Geometry check sheet. Reference: the model listing, model coordinates, mm. A direction names the side the tool comes from. Coordinates: 2 decimals unless noted, no trailing zeros. Loops run counter-clockwise (first coordinate to the right, second up) from the corner with the lowest first, then second, coordinate; pieces in that order, holes last. Notation, with made-up numbers: (-7.5, 81) - (47.5, 81) arc R19 ccw to (47.5, 92) - close; hole circle Ø9 at (4, -9). An arc over 180 degrees is marked (long way). Write each question's results on one line, items separated by ' | '. Start each with the question number.
(1) Material ranges on probe 1 along Y at (x, z) = (0, 6); probe 2 along Y at (x, z) = (0.5, 10.25); probe 3 along X at (y, z) = (-8, 2), recorded low to high.
(2) Sectioned sample at A-A (y = 0). Enter the section's corners in (x, z).
(3) Sectioned sample at B-B (x = 0). Enter the section's corners in (y, z).
(4) Mould release check, pull along X, two halves, no side actions. Record for faces 3 (the face through (10.4, -1.2, 5.6)), 4 (the face through (-6, 17, 0.95)), 5 (the face through (4.119, 18.548, 0.468)): pulls with the +X half, pulls with the -X half, needs draft (parallel to the pull), parting line crosses it, or undercut.
(5) Access from +Z, -Z, +X, -X, +Y, -Y to the whole of each face (thin tool, end or side, straight path). Record for faces 1 (the face through (12.384, 5.419, 5.552)), 2 (the face through (-13.887, -10.648, 5.88)).
(6) Sectioned sample at C-C (y = 4). Enter the section's corners in (x, z).
(7) Sectioned sample at D-D (x = -12.5). Enter the section's corners in (y, z).
(8) Go/stop test with flat-tipped pins: pin 1 Ø11 at (x, y) = (0, 0) entering from -Z; pin 2 Ø6 at (x, z) = (9.5, 2) entering from +Y; pin 3 Ø1.5 at (y, z) = (0.5, 5.5) entering from +X; pin 4 Ø3 at (y, z) = (15, 6.5) entering from +X. Record where each tip stops, or that it passes through.
from build123d import *

# Parameters (mm, degrees)
SKETCH_1_R          = 17.5
EXTRUDE_1_DEPTH     = 10.95
SKETCH_1_4_R        = 19
SKETCH_1_4_R_2      = 17.5
EXTRUDE_2_DEPTH     = 0.95
SKETCH_2_R          = 9
SKETCH_2_R_2        = 1.5
SKETCH_2_R_3        = 2
CUT_EXTRUDE_1_DEPTH = 30.015556173


with BuildPart() as part:
    # Sketch 1 → Extrude 1 (new body)
    with BuildSketch(Plane.XY):
        Circle(SKETCH_1_R)
    extrude(amount=EXTRUDE_1_DEPTH)

    # Sketch 1_4 → Extrude 2 (add)
    with BuildSketch(Plane.XY):
        with Locations(Location((0, 0, 0), (0, 0, 180))):
            Circle(SKETCH_1_4_R)
        Circle(SKETCH_1_4_R_2, mode=Mode.SUBTRACT)
    extrude(amount=EXTRUDE_2_DEPTH)

    # Sketch 2 → Cut-Extrude 1 (cut, through all)
    with BuildSketch(Plane.XY.offset(10.95)):
        Circle(SKETCH_2_R)
        with Locations((0, 13.5)):
            Circle(SKETCH_2_R_2)
        with Locations((11.691342951, 6.75)):
            Circle(SKETCH_2_R_2)
        with Locations((11.691342951, -6.75)):
            Circle(SKETCH_2_R_2)
        with Locations((0, -13.5)):
            Circle(SKETCH_2_R_2)
        with Locations((-11.691342951, -6.75)):
            Circle(SKETCH_2_R_2)
        with Locations((-11.691342951, 6.75)):
            Circle(SKETCH_2_R_2)
        with Locations((12, 0)):
            Circle(SKETCH_2_R_3)
        with Locations((-6, -10.392304845)):
            Circle(SKETCH_2_R_3)
        with Locations((-6, 10.392304845)):
            Circle(SKETCH_2_R_3)
    extrude(amount=-CUT_EXTRUDE_1_DEPTH, mode=Mode.SUBTRACT)


solid = part.part
Outcome:
1) probe 1: y = -17.5 to -15, -12 to -9, 9 to 12, 15 to 17.5 | probe 2: y = -17.49 to -14.91, -12.09 to -8.99, 8.99 to 12.09, 14.91 to 17.49 | probe 3: x = -15.56 to -12.52, -10.86 to -4.12, 4.12 to 10.86, 12.52 to 15.56
2) outline: (-19, 0) - (-9, 0) - (-9, 10.95) - (-17.5, 10.95) - (-17.5, 0.95) - (-19, 0.95) - close; (9, 0) - (10, 0) - (10, 10.95) - (9, 10.95) - close; (14, 0) - (19, 0) - (19, 0.95) - (17.5, 0.95) - (17.5, 10.95) - (14, 10.95) - close
3) outline: (-19, 0) - (-15, 0) - (-15, 10.95) - (-17.5, 10.95) - (-17.5, 0.95) - (-19, 0.95) - close; (-12, 0) - (-9, 0) - (-9, 10.95) - (-12, 10.95) - close; (9, 0) - (12, 0) - (12, 10.95) - (9, 10.95) - close; (15, 0) - (19, 0) - (19, 0.95) - (17.5, 0.95) - (17.5, 10.95) - (15, 10.95) - close
4) face 3: undercut | face 4: needs draft | face 5: parting line crosses it
5) face 1: +Z, -Z | face 2: +Z
6) outline: (-18.57, 0) - (-8.06, 0) - (-8.06, 10.95) - (-17.04, 10.95) - (-17.04, 0.95) - (-18.57, 0.95) - close; (8.06, 0) - (18.57, 0) - (18.57, 0.95) - (17.04, 0.95) - (17.04, 10.95) - (8.06, 10.95) - close
7) outline: (-14.31, 0) - (-8.01, 0) - (-8.01, 10.95) - (-12.25, 10.95) - (-12.25, 0.95) - (-14.31, 0.95) - close; (-5.49, 0) - (5.49, 0) - (5.49, 10.95) - (-5.49, 10.95) - close; (8.01, 0) - (14.31, 0) - (14.31, 0.95) - (12.25, 0.95) - (12.25, 10.95) - (8.01, 10.95) - close
8) pin 1: passes through | pin 2: stops at y = 17.78 | pin 3: stops at x = 17.5 | pin 4: stops at x = 11.14
